Could you check a few things on this model? Use its own coordinates, in mm. A direction names the side the tool comes from. Round coordinates to 2 decimals unless told otherwise and drop trailing zeros. Loops run counter-clockwise (first coordinate to the right, second up) from the corner with the lowest first, then second, coordinate; pieces in that order, holes last. Notation, with made-up numbers: (44, -40) -> (68, -40) arc R24 cw to (68, -2) -> close; hole circle Ø4 at (5.5, 10). An arc over 180 degrees is marked (long way). One line per item, written item: value.
```python
from build123d import *

# Parameters (mm, degrees)
PAD_DEPTH           = 2
FILLET_R            = 0.2
SKETCH001_W         = 6.9
SKETCH001_H         = 0.8
POCKET_DEPTH        = 0.5
SKETCH002_W         = 0.95
SKETCH002_H         = 1.3
POCKET001_DEPTH     = 0.2
SKETCH003_W         = 2
SKETCH003_H         = 1.5
POCKET002_DEPTH     = 0.25
SKETCH004_W         = 6.9
SKETCH004_H         = 0.25
POCKET003_DEPTH     = 0.75
SKETCH005_W         = 4.4
SKETCH005_H         = 0.7
POCKET004_DEPTH     = 0.25
PAD001_DEPTH        = 2.7
FILLET001_R         = 0.2
SKETCH007_W         = 0.37
SKETCH007_H         = 0.25
POCKET005_DEPTH     = 2.7
LINEARPATTERN_COUNT = 5
LINEARPATTERN_PITCH = 0.65


with BuildPart() as part:
    # Sketch → Pad (new body)
    with BuildSketch(Plane.XY):
        Polygon((-3.45, 1), (3.45, 1), (3.45, 0.25), (2.45, -1.1), (-2.45, -1.1), (-3.45, 0.25), align=None)
    extrude(amount=PAD_DEPTH)

    # Fillet
    fillet_edges = [part.edges().sort_by_distance(p)[0] for p in [
        (3.45, 1, 1),
        (3.45, 0.25, 1),
        (2.45, -1.1, 1),
        (-2.45, -1.1, 1),
        (-3.45, 0.25, 1),
        (-3.45, 1, 1),
    ]]
    fillet(fillet_edges, radius=FILLET_R)

    # Sketch001 (on Face5 of Fillet) → Pocket (cut)
    with BuildSketch(Plane.XY.offset(2)):
        with Locations((0, -0.7)):
            Rectangle(SKETCH001_W, SKETCH001_H)
    extrude(amount=-POCKET_DEPTH, mode=Mode.SUBTRACT)

    # Sketch002 (on Face4 of Pocket) → Pocket001 (cut)
    with BuildSketch(Plane.XY.offset(2)):
        with Locations((-2.975, 0.35)):
            Rectangle(SKETCH002_W, SKETCH002_H)
        with Locations((2.975, 0.35)):
            Rectangle(SKETCH002_W, SKETCH002_H)
    extrude(amount=-POCKET001_DEPTH, mode=Mode.SUBTRACT)

    # Sketch003 (on Face8 of Pocket001) → Pocket002 (cut)
    with BuildSketch(Plane.XZ.offset(1.1)):
        with Locations((0, 0.75)):
            Rectangle(SKETCH003_W, SKETCH003_H)
    extrude(amount=-POCKET002_DEPTH, mode=Mode.SUBTRACT)

    # Sketch004 (on Face2 of Pocket002) → Pocket003 (cut)
    with BuildSketch(Plane(origin=(0, 0, 0), x_dir=(1, 0, 0), z_dir=(0, 0, -1))):
        with Locations((0, 0.975)):
            Rectangle(SKETCH004_W, SKETCH004_H)
    extrude(amount=-POCKET003_DEPTH, mode=Mode.SUBTRACT)

    # Sketch005 (on Face12 of Pocket003) → Pocket004 (cut)
    with BuildSketch(Plane(origin=(0, 1, 0), x_dir=(-1, 0, 0), z_dir=(0, 1, 0))):
        with Locations((0, 1.4)):
            Rectangle(SKETCH005_W, SKETCH005_H)
    extrude(amount=-POCKET004_DEPTH, mode=Mode.SUBTRACT)

    # Sketch006 (on Face2 of Pocket004) → Pad001 (join)
    with BuildSketch(Plane(origin=(0, 0, 0), x_dir=(1, 0, 0), z_dir=(0, 0, -1))):
        with BuildLine():
            Line((-1.55, -0.15), (1.55, -0.15))
            ThreePointArc((1.750006, -0.35), (1.691425, -0.208577), (1.55, -0.15))
            Line((1.750006, -0.35), (1.750006, -0.55))
            ThreePointArc((1.550006, -0.75), (1.691427, -0.691421), (1.750006, -0.55))
            Line((1.550006, -0.75), (-1.549994, -0.75))
            ThreePointArc((-1.749994, -0.55), (-1.691416, -0.691421), (-1.549994, -0.75))
            Line((-1.749994, -0.35), (-1.749994, -0.55))
            ThreePointArc((-1.55, -0.15), (-1.691418, -0.208581), (-1.749994, -0.35))
        make_face()
    extrude(amount=PAD001_DEPTH)

    # Fillet001
    fillet001_edges = [part.edges().sort_by_distance(p)[0] for p in [
        (-1.691418, 0.208581, -2.7),
        (0, 0.15, -2.7),
        (1.691425, 0.208577, -2.7),
        (1.750006, 0.45, -2.7),
        (1.691427, 0.691421, -2.7),
        (6e-06, 0.75, -2.7),
        (-1.691416, 0.691421, -2.7),
        (-1.749994, 0.45, -2.7),
    ]]
    fillet(fillet001_edges, radius=FILLET001_R)

    # Sketch007 (on Face8 of Fillet001) → Pocket005 (cut)
    with BuildSketch(Plane(origin=(0, 0, -2.7), x_dir=(1, 0, 0), z_dir=(0, 0, -1))):
        with Locations((-1.3, -0.275)):
            Rectangle(SKETCH007_W, SKETCH007_H)
    pocket005 = extrude(amount=-POCKET005_DEPTH, mode=Mode.SUBTRACT)

    # LinearPattern: Pocket005 ×5
    with Locations(*[(i * LINEARPATTERN_PITCH, 0, 0) for i in range(1, LINEARPATTERN_COUNT)]):
        add(pocket005, mode=Mode.SUBTRACT)


solid = part.part
```
(1) Imagine slicing it at A-A on z = 1.3. Write out the boundary of the cut face in (x, y), then the cut area to 3 significant figures.
Results below:
outline: (-3.45, 0.32) arc R0.2 ccw to (-3.41, 0.2) -> (-2.51, -1.02) arc R0.2 ccw to (-2.35, -1.1) -> (-1, -1.1) -> (-1, -0.85) -> (1, -0.85) -> (1, -1.1) -> (2.35, -1.1) arc R0.2 ccw to (2.51, -1.02) -> (3.41, 0.2) arc R0.2 ccw to (3.45, 0.32) -> (3.45, 0.8) arc R0.2 ccw to (3.25, 1) -> (2.2, 1) -> (2.2, 0.75) -> (-2.2, 0.75) -> (-2.2, 1) -> (-3.25, 1) arc R0.2 ccw to (-3.45, 0.8) -> close
area: 11.5 mm²
(2) Please list where these lines run through material, in increasing order: L1, parallel to Z at x = 2.25, y = 0.45; L2, parallel to Z at x = -1, y = -0.7; L3, parallel to Z at x = -0.25, y = 0.95.
Results below:
L1: z = 0 to 2
L2: z = 0 to 1.5
L3: z = 0 to 1.05, 1.75 to 2
(3) We'd pull the mould along X, two halves only. Please class faces 5 (the face through (-3, 0, 1.8)), 6 (the face through (-2.954, -0.42, 0.887)), 7 (the face through (0, -0.85, 1)), 8 (the face through (2.97, -0.4, 0.89)): +X half, -X half, draft (parallel to the pull), parting line (faces both ways), or undercut.
Results below:
face 5: draft
face 6: -X half
face 7: undercut
face 8: +X half
(4) On a 3-axis mill with a long thin cutter (end or side, diameter ignored), from which of +Z, -Z, +X, -X, +Y, -Y can I reach the whole of each face in a straight line? I mean faces 1 (the face through (0, 0.75, -1)), 2 (the face through (3, 0, 1.8)), 3 (the face through (0, -0.6, 1.5)), 4 (the face through (0, 0, 2)). Say none if no direction works.
Results below:
face 1: -Z, +X, -X, +Y
face 2: +Z, +X, +Y, -Y
face 3: +Z, +X, -X, -Y
face 4: +Z, +X, -X, +Y, -Y
(5) Imagine slicing it at D-D on z = 0.2. Write out the boundary of the cut face in (x, y).
Results below:
outline: (-3.45, 0.32) arc R0.2 ccw to (-3.41, 0.2) -> (-2.64, -0.85) -> (2.64, -0.85) -> (3.41, 0.2) arc R0.2 ccw to (3.45, 0.32) -> (3.45, 0.8) arc R0.2 ccw to (3.25, 1) -> (-3.25, 1) arc R0.2 ccw to (-3.45, 0.8) -> close
(6) Imagine slicing it at B-B on x = 1.25. Write out the boundary of the cut face in (y, z), then the cut area to 3 significant figures.
Results below:
outline: (-1.1, 0.75) -> (-0.85, 0.75) -> (-0.85, 0) -> (0.4, 0) -> (0.4, -2.7) -> (0.55, -2.7) arc R0.2 ccw to (0.75, -2.5) -> (0.75, 0) -> (1, 0) -> (1, 1.05) -> (0.75, 1.05) -> (0.75, 1.75) -> (1, 1.75) -> (1, 2) -> (-0.3, 2) -> (-0.3, 1.5) -> (-1.1, 1.5) -> close
area: 4.37 mm²
(7) Imagine slicing it at C-C on y = -0.05. Write out the boundary of the cut face in (x, z).
Results below:
outline: (-3.23, 0) -> (3.23, 0) -> (3.23, 1.8) -> (2.5, 1.8) -> (2.5, 2) -> (-2.5, 2) -> (-2.5, 1.8) -> (-3.23, 1.8) -> close
